Answer from the drawing. Dimensions are ordinates in mm from the lowest x, y and z of the part. A direction names the side the tool comes from. Coordinates: 2 decimals unless noted, no trailing zeros. Write each loop counter-clockwise with the first axis right and the second up, starting at its lowest first coordinate (ties: lowest second). Pieces come first, ordered by that corner, then holes. Notation, with made-up numbers: (65, -33.75) - (106, -33.75) arc R25 cw to (106, -4.75) - close; hole circle Ø6 at (74, 23.5). An arc over 180 degrees is marked (long way). Use one line per item in the form item = value. Start each with the question number.
Item 1: For the marked faces 4 and 5, determine the directions among +Z, -Z, +X, -X, +Y, -Y from which every point of the face is accessible in a straight line to the end or side of a thin tool.
Item 2: Determine the mould class of the marked faces 1, 2 and 3 for opening direction Y: released by +Y, released by -Y, zero draft, split by the parting line, or undercut.
Item 3: A cutting plane is placed at C-C (x = 44.5). Write down the section's boundary in (y, z).
Item 4: Given pin 1 (8.5 mm diameter, centred on x = 75, y = 8.5, fed in from +Z); pin 2 (2 mm diameter, centred on y = 39.5, z = 11.5, fed in from -X); pin 3 (16 mm diameter, centred on x = 77, z = 31, fed in from -Y); pin 4 (1.5 mm diameter, centred on x = 59, y = 97, fed in from -Z), each flat-ended and moving along its own axis, determine where each tip first touches the part or whether it passes through.
Item 5: A cutting plane is placed at B-B (z = 29.5). Write down the section's boundary in (x, y).
Item 6: A cutting plane is placed at D-D (y = 53). Write down the section's boundary in (x, z).
Item 7: A cutting plane is placed at A-A (y = 8.5). Write down the section's boundary in (x, z), then the cut area to 3 significant figures.
Item 8: Consider probe 1 along Y at (x, z) = (75, 1.9); probe 2 along X at (y, z) = (33, 27.5); probe 3 along X at (y, z) = (17.5, 45). Determine where each line is inside the solid, lowest interval first.
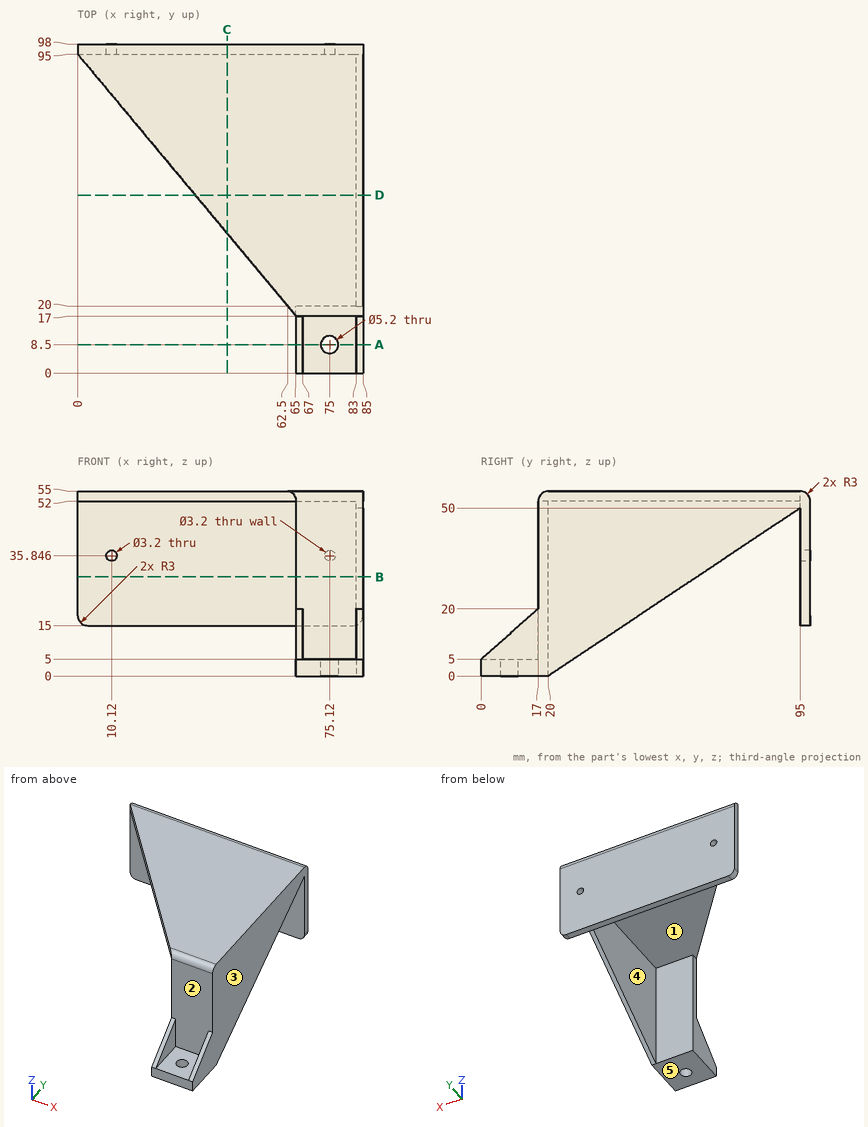
Answer:
q1.face_4 = -Z, -X
q1.face_5 = -Z, +X, -X, +Y, -Y
q2.face_1 = undercut
q2.face_2 = released by -Y
q2.face_3 = zero draft
q3.outline = (41.6, 52) - (95, 52) - (95, 15) - (98, 15) - (98, 52) arc R3 ccw to (95, 55) - (41.6, 55) - close
q4.pin_1 = 5
q4.pin_2 = through
q4.pin_3 = 17
q4.pin_4 = 15
q5.outline = (0, 95) - (85, 95) - (85, 98) - (0, 98) - close; (65, 17) - (85, 17) - (85, 64.25) - (83, 64.25) - (83, 20) - (65, 20) - close
q6.outline = (35, 52) - (83, 52) - (83, 22) - (85, 22) - (85, 55) - (35, 55) - close
q7.outline = (65, 0) - (72.4, 0) - (72.4, 5) - (67, 5) - (67, 12.5) - (65, 12.5) - close; (77.6, 0) - (85, 0) - (85, 12.5) - (83, 12.5) - (83, 5) - (77.6, 5) - close
q7.area = 104 mm²
q8.probe_1 = 0 to 5.9, 11.1 to 20
q8.probe_2 = 83 to 85
q8.probe_3 = 65 to 85
